Here's how the part is built. I have some questions about the finished solid (model axes, mm). A direction names the side the tool comes from. Round coordinates to 2 decimals unless told otherwise and drop trailing zeros. Loops run counter-clockwise (first coordinate to the right, second up) from the corner with the lowest first, then second, coordinate; pieces in that order, holes last. Notation, with made-up numbers: M 6,-32.5 L 30,-32.5 A15 cw 30,-23.5 Z; hole C 71.25,50 d6. An arc over 180 degrees is marked long. Use a Markdown table: item, result.
from build123d import *

# Parameters (mm, degrees)
BOX043_W               = 14
BOX043_H               = 73
BOX043_DEPTH           = 51
BOX043_PLACEMENT_ANGLE = 15
CYLINDER122_R          = 2.6
CYLINDER122_DEPTH      = 47
CYLINDER117_R          = 6
CYLINDER117_DEPTH      = 40
CYLINDER118_R          = 2.1
CYLINDER118_DEPTH      = 10
CYLINDER119_R          = 6
CYLINDER119_DEPTH      = 40
CYLINDER120_R          = 2.1
CYLINDER120_DEPTH      = 10
CYLINDER121_R          = 18
CYLINDER121_DEPTH      = 13
EXTRUDE035_DEPTH       = 30


with BuildPart() as box043:
    # Box043 → Box043 (new body)
    with BuildSketch(Plane.XY):
        with Locations((7, 36.5)):
            Rectangle(BOX043_W, BOX043_H)
    extrude(amount=BOX043_DEPTH)


with BuildPart() as box043_1:
    # Box043 placement: moved
    add(box043.part.moved(Location((336.936297, -53.3, -1.035276))).rotate(Axis((336.936297, -53.3, -1.035276), (0, -1, 0)), BOX043_PLACEMENT_ANGLE))


with BuildPart() as cylinder122:
    # Cylinder122 → Cylinder122 (new body)
    with BuildSketch(Plane(origin=(316, 5.5, 32.2), x_dir=(1, 0, 0), z_dir=(0, -1, 0))):
        Circle(CYLINDER122_R)
    extrude(amount=CYLINDER122_DEPTH)


with BuildPart() as cylinder117:
    # Cylinder117 → Cylinder117 (new body)
    with BuildSketch(Plane.XY.offset(10)):
        Circle(CYLINDER117_R)
    extrude(amount=CYLINDER117_DEPTH)


with BuildPart() as fusion056:
    # Cylinder118 → Cylinder118 (new body)
    with BuildSketch(Plane.XY):
        Circle(CYLINDER118_R)
    extrude(amount=CYLINDER118_DEPTH)

    # Fusion056: union Cylinder117
    add(cylinder117.part)


with BuildPart() as fusion056_1:
    # Fusion056 placement: moved
    add(fusion056.part.moved(Location((322, 5, -5))))


with BuildPart() as cylinder119:
    # Cylinder119 → Cylinder119 (new body)
    with BuildSketch(Plane.XY.offset(10)):
        Circle(CYLINDER119_R)
    extrude(amount=CYLINDER119_DEPTH)


with BuildPart() as fusion057:
    # Cylinder120 → Cylinder120 (new body)
    with BuildSketch(Plane.XY):
        Circle(CYLINDER120_R)
    extrude(amount=CYLINDER120_DEPTH)

    # Fusion057: union Cylinder119
    add(cylinder119.part)


with BuildPart() as fusion057_1:
    # Fusion057 placement: moved
    add(fusion057.part.moved(Location((322, -41, -5))))


with BuildPart() as cylinder121:
    # Cylinder121 → Cylinder121 (new body)
    with BuildSketch(Plane(origin=(313, -11, 35), x_dir=(1, 0, 0), z_dir=(0, -1, 0))):
        Circle(CYLINDER121_R)
    extrude(amount=CYLINDER121_DEPTH)


with BuildPart() as cut108:
    # Sketch028 → Extrude035 (new body)
    with BuildSketch(Plane.YZ):
        Polygon((15, 0), (-49.79, 0), (-49.79, 12), (-27.183378, 42), (-7.606622, 42), (15, 12), align=None)
    extrude(amount=-EXTRUDE035_DEPTH)


with BuildPart() as cut108_1:
    # Extrude035 placement: moved
    add(cut108.part.moved(Location((337, 0, 0))))

    # Cut104: cut Cylinder121
    add(cylinder121.part, mode=Mode.SUBTRACT)

    # Cut105: cut Fusion057
    add(fusion057_1.part, mode=Mode.SUBTRACT)

    # Cut106: cut Fusion056
    add(fusion056_1.part, mode=Mode.SUBTRACT)

    # Cut107: cut Cylinder122
    add(cylinder122.part, mode=Mode.SUBTRACT)

    # Cut108: cut Box043
    add(box043_1.part, mode=Mode.SUBTRACT)


with BuildPart() as cut108_2:
    # Cut108 placement: moved
    add(cut108_1.part.moved(Location((0, 41.7, 0))))


solid = cut108_2.part
1. Imagine slicing it at D-D, the plane x = 310.75. Write out the boundary of the cut face in (y, z), then the cut area to 3 significant figures.
Answer sheet:
| item | result |
|---|---|
| outline | M -8.09,0 L 56.7,0 L 56.7,12 L 34.09,42 L 30.7,42 L 30.7,17.14 L 17.7,17.14 L 17.7,42 L 14.52,42 L -8.09,12 Z |
| area | 1,720 mm2 |
2. Imagine slicing it at C-C, the plane z = 30.5. Write out the boundary of the cut face in (x, y).
Answer sheet:
| item | result |
|---|---|
| outline | M 307,5.85 L 314.03,5.85 L 314.03,17.7 L 307,17.7 Z; M 307,30.7 L 314.03,30.7 L 314.03,42.76 L 307,42.76 Z; M 317.97,5.85 L 318.92,5.85 A6 cw 325.08,5.85 L 328.49,5.85 L 328.49,17.7 L 317.97,17.7 Z; M 317.97,30.7 L 328.49,30.7 L 328.49,42.76 L 326.52,42.76 A6 cw 317.97,42.26 Z |
3. I need wall thicknesses on probe 1 along Y at (x, z) = (322, 2.8); probe 2 along Z at (x, y) = (317.75, 48.5); probe 3 along Y at (x, z) = (319.5, 37). Which ranges of each line are inside material? Lowest first, please. Write a range as from..to.
Answer sheet:
| item | result |
|---|---|
| probe 1 | -8.09..-1.4, 2.8..44.6, 48.8..56.7 |
| probe 2 | 0..5 |
| probe 3 | 10.75..17.7, 30.7..37.86 |
4. We'd pull the mould along Y, two halves only. Please class faces 3 (the face through (322, 56.7, 6)), 4 (the face through (319.9, 46.79, 2.46)), 5 (the face through (332.36, 23.85, 16.04)): +Y half, -Y half, draft (parallel to the pull), parting line (faces both ways), or undercut.
Answer sheet:
| item | result |
|---|---|
| face 3 | +Y half |
| face 4 | undercut |
| face 5 | draft |
5. Which directions (+Z, -Z, +X, -X, +Y, -Y) give clear straight access to the entire face, cutting with the end or side of a thin tool? Please do faces 1 (the face through (322, -2, 5)), 2 (the face through (316, 16, 42)).
Answer sheet:
| item | result |
|---|---|
| face 1 | +Z |
| face 2 | +Z, +X, -X, +Y, -Y |
6. Imagine slicing it at A-A, the plane x = 322. Write out the boundary of the cut face in (y, z), then the cut area to 3 significant figures.
Answer sheet:
| item | result |
|---|---|
| outline | M -8.09,0 L -1.4,0 L -1.4,5 L -5.3,5 L -5.3,15.7 L -8.09,12 Z; M 2.8,0 L 44.6,0 L 44.6,5 L 40.7,5 L 40.7,33.23 L 34.09,42 L 30.7,42 L 30.7,19.41 L 17.7,19.41 L 17.7,42 L 14.52,42 L 6.7,31.63 L 6.7,5 L 2.8,5 Z; M 48.8,0 L 56.7,0 L 56.7,12 L 52.7,17.31 L 52.7,5 L 48.8,5 Z |
| area | 1,240 mm2 |
7. For pin 1 Ø2 at (x, z) = (329.5, 16.5) entering from -Y; pin 2 Ø9.5 at (x, y) = (319, 1.5) entering from +Z; pin 3 Ø6.5 at (x, z) = (317.5, 33.5) entering from -Y, each with a flat end and sliding along its axis, tell me the tip position at first contact or that it passes through.
Answer sheet:
| item | result |
|---|---|
| pin 1 | y = -5.45 |
| pin 2 | z = 31.03 |
| pin 3 | y = 5.67 |
8. Imagine slicing it at B-B, the plane y = 46.7. Write out the boundary of the cut face in (x, z), then the cut area to 3 significant figures.
Answer sheet:
| item | result |
|---|---|
| outline | M 307,0 L 319.9,0 L 319.9,5 L 316,5 L 316,25.27 L 307,25.27 Z; M 324.1,0 L 336.66,0 L 329.89,25.27 L 328,25.27 L 328,5 L 324.1,5 Z |
| area | 400 mm2 |
